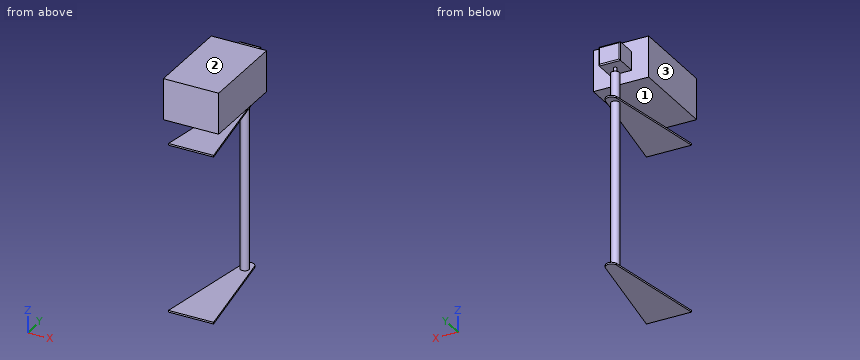
Autodesk Inventor part; units mm, degrees
ref_plane "YZ Plane" through (0, 0, 0) normal (1, 0, 0) x (0, 1, 0)
ref_plane "XZ Plane" through (0, 0, 0) normal (0, 1, 0) x (-1, 0, 0)
ref_plane "XY Plane" through (0, 0, 0) normal (0, 0, 1) x (1, 0, 0)
sketch "Sketch1" plane through (0, 0, 0) normal (0, 0, 1) x (1, 0, 0)
  point P0 (0, 0)
sketch "Sketch2" plane through (0, 0, 0) normal (0, 0, 1) x (1, 0, 0)
  line L0 (0, 0) -> (80, 0)
  line L1 (80, 0) -> (40, 250)
  line L2 (40, 250) -> (0, 0)
  dimension "d0" = 80
  dimension "d1" = 250
  dimension "d2" = 40
extrude "Extrusion1" add sketch "Sketch2" against normal blind 3
sketch "Sketch3" plane through (0, 0, -3) normal (0, 0, -1) x (-1, 0, 0)
  circle A0 centre (-40, 175) radius 7.5
  line L0 (-80, 0) -> (0, 0)
  point P0 (-40, 250)
  point P1 (-40, 0)
  dimension "d5" = 15
  dimension "d6" = 0
  dimension "d7" = 175
fillet "Fillet1" radius 10 1 edges at (40, 250, -1.5)
extrude "Extrusion2" add sketch "Sketch3" along normal blind 147
mirror "Mirror1" about plane through (40, 175, -150) normal (0, 0, -1) of "Extrusion2", "Extrusion1"
fillet "Fillet2" radius 10 1 edges at (40, 250, -298.5)
sketch "Sketch4" plane through (0, 0, 0) normal (0, 0, 1) x (1, 0, 0)
  circle A0 centre (40, 175) radius 7.5
  circle A1 centre (40, 175) radius 7.5
  point P0 (0, 0)
extrude "Extrusion3" add sketch "Sketch4" along normal blind 50
sketch "Sketch5" plane through (40, 175, 50) normal (0, 0, 1) x (1, 0, 0)
  circle A0 centre (0, 0) radius 2.5
  point P0 (-40, -175)
  dimension "d14" = 5
extrude "Extrusion4" add sketch "Sketch5" along normal blind 10
sketch "Sketch6" plane through (40, 175, 60) normal (0, 0, 1) x (1, 0, 0)
  line L0 (-19, 19) -> (19, 19)
  line L1 (19, 19) -> (19, -19)
  line L2 (19, -19) -> (-19, -19)
  line L3 (-19, -19) -> (-19, 19)
  circle A0 centre (0, 0) radius 2.5
  point P0 (-40, -175)
  dimension "d17" = 38
  dimension "d18" = 38
  dimension "d19" = 19
  dimension "d20" = 19
extrude "Extrusion5" add sketch "Sketch6" along normal blind 33 contours L0 L1 L2 L3 | A0
sketch "Sketch7" plane through (21, 156, 60) normal (0, -1, 0) x (1, 0, 0)
  line L0 (-30, 53) -> (68, 53)
  line L1 (68, 53) -> (68, -20)
  line L2 (68, -20) -> (-30, -20)
  line L3 (-30, -20) -> (-30, 53)
  line L4 (38, 0) -> (38, 33)
  line L5 (0, 0) -> (0, 33)
  line L6 (0, 33) -> (38, 33)
  point P0 (-21, -60)
  point P1 (38, 16.5)
  point P2 (68, 16.5)
  point P3 (-30, 16.5)
  point P4 (0, 16.5)
  dimension "d23" = 30
  dimension "d24" = 30
  dimension "d25" = 20
  dimension "d26" = 20
extrude "Extrusion6" add sketch "Sketch7" along normal blind 156
fillet "Fillet3" radius 2 4 edges at (21, 194, 76.5) (59, 194, 76.5) (40, 194, 60) (40, 194, 93)
properties part number "stand"
For this review, take the finished solid that the model builds, in its own axes (mm). Face numbers are marked on the shaded views. Coordinates: 2 decimals unless noted, no trailing zeros. Write each loop counter-clockwise with the first axis right and the second up, starting at its lowest first coordinate (ties: lowest second). Pieces come first, ordered by that corner, then holes. Notation, with made-up numbers: (-8.5, -21.5) -> (-4.5, -21.5) arc R12 cw to (-4.5, -0.5) -> close; hole circle Ø11 at (-3.5, -2). An arc over 180 degrees is marked (long way). Write each question's results on one line, items separated by ' | '. Start each with the question number.
1) Consider section B-B (x = 70). Write out the cut boundary in (y, z), plus the area to 3 significant figures.
2) The part is to be moulded in two halves that separate along Z. For the marked faces 1, 2 and 3, say which applies: +Z half, -Z half, draft (parallel to the pull), parting line (faces both ways), or undercut.
3) Insertion check: pin 1 (14.5 mm diameter, centred on x = 36, z = 71.5, fed in from +Y); pin 2 (2 mm diameter, centred on x = 15, y = 94.5, fed in from -Z); pin 3 (10 mm diameter, centred on y = 179, z = 80.5, fed in from +X); pin 4 (6 mm diameter, centred on x = 71.5, y = 156, fed in from -Z). Each pin has a flat end and moves straight along its axis. Give the tip position at first contact, or say it passes through.
4) Consider section A-A (y = 84). Write out the cut boundary in (x, z).
5) Consider section C-C (z = -262). Write out the cut boundary in (x, y).
6) Wall thickness on L1, parallel to Z at x = 39.5, y = 136.5; L2, parallel to Z at x = 18, y = 147; L3, parallel to Y at x = 9, z = 78: over which ranges is each line inside the solid? List them lowest first. Write a range as [from, to].
Geometry says:
1) outline: (0, -300) -> (62.5, -300) -> (62.5, -297) -> (0, -297) -> close; (0, -3) -> (62.5, -3) -> (62.5, 0) -> (0, 0) -> close; (0, 40) -> (156, 40) -> (156, 113) -> (0, 113) -> close | area: 11,800 mm^2
2) face 1: undercut | face 2: +Z half | face 3: draft
3) pin 1: y = 194 | pin 2: z = -300 | pin 3: x = 59 | pin 4: z = 40
4) outline: (-9, 40) -> (89, 40) -> (89, 113) -> (-9, 113) -> close; (13.44, -300) -> (66.56, -300) -> (66.56, -297) -> (13.44, -297) -> close; (13.44, -3) -> (66.56, -3) -> (66.56, 0) -> (13.44, 0) -> close
5) outline: circle Ø15 at (40, 175)
6) L1: [-300, -297], [-3, 0], [40, 113] | L2: [40, 113] | L3: [0, 156]
